from build123d import *

# Parameters (mm, degrees)
BOSS_EXTRUDE1_DEPTH = 2
SKETCH2_W           = 10
SKETCH2_H           = 30
CUT_EXTRUDE1_DEPTH  = 3
FILLET1_R           = 1
CUT_EXTRUDE2_REACH  = 4
SKETCH3_R           = 1.6


with BuildPart() as part:
    # Sketch1 → Boss-Extrude1 (new body)
    with BuildSketch(Plane(origin=(0, 0, 0), x_dir=(1, 0, 0), z_dir=(0, 1, 0))):
        with BuildLine():
            ThreePointArc((-49.7, -34.741676707), (-48.154415588, -35.654415588), (-47.241676707, -37.2))
            Line((-47.241676707, -37.2), (47.241676707, -37.2))
            ThreePointArc((47.241676707, -37.2), (48.154415588, -35.654415588), (49.7, -34.741676707))
            Line((49.7, -34.741676707), (49.7, 34.741676707))
            ThreePointArc((49.7, 34.741676707), (48.154415588, 35.654415588), (47.241676707, 37.2))
            Line((47.241676707, 37.2), (-47.241676707, 37.2))
            ThreePointArc((-47.241676707, 37.2), (-48.154415588, 35.654415588), (-49.7, 34.741676707))
            Line((-49.7, 34.741676707), (-49.7, -34.741676707))
        make_face()
    extrude(amount=BOSS_EXTRUDE1_DEPTH)

    # Sketch2 → Cut-Extrude1 (cut, through all)
    with BuildSketch(Plane(origin=(0, 2, 0), x_dir=(1, 0, 0), z_dir=(0, 1, 0))):
        with Locations((-34.7, 0)):
            Rectangle(SKETCH2_W, SKETCH2_H)
    extrude(amount=-CUT_EXTRUDE1_DEPTH, mode=Mode.SUBTRACT)

    # Fillet1
    fillet1_edges = [part.edges().sort_by_distance(p)[0] for p in [
        (-29.7, 1, -15),
        (-29.7, 1, 15),
        (-39.7, 1, 15),
        (-39.7, 1, -15),
    ]]
    fillet(fillet1_edges, radius=FILLET1_R)

    # Sketch3 → Cut-Extrude2 (cut, up to next)
    with BuildSketch(Plane(origin=(0, 2, 0), x_dir=(1, 0, 0), z_dir=(0, 1, 0)), mode=Mode.PRIVATE) as cut_extrude2_sk1:
        with Locations((-13.794673406, 16.290721811)):
            Circle(SKETCH3_R)
    cut_extrude2_tool1 = extrude(cut_extrude2_sk1.sketch, amount=-CUT_EXTRUDE2_REACH, mode=Mode.PRIVATE) & part.part
    add(cut_extrude2_tool1.solids().sort_by_distance((-13.794673, 2, -16.290722))[0], mode=Mode.SUBTRACT)
    # Sketch3 → Cut-Extrude2 (cut, up to next)
    with BuildSketch(Plane(origin=(0, 2, 0), x_dir=(1, 0, 0), z_dir=(0, 1, 0)), mode=Mode.PRIVATE) as cut_extrude2_sk2:
        with Locations((34.973326594, -9.541278189)):
            Circle(SKETCH3_R)
    cut_extrude2_tool2 = extrude(cut_extrude2_sk2.sketch, amount=-CUT_EXTRUDE2_REACH, mode=Mode.PRIVATE) & part.part
    add(cut_extrude2_tool2.solids().sort_by_distance((34.973327, 2, 9.541278))[0], mode=Mode.SUBTRACT)


solid = part.part
For this review, take the finished solid that the model builds, in its own axes (mm). A direction names the side the tool comes from. Give positions to 0.01 mm unless a question says otherwise; leave off trailing zeros. Loops run counter-clockwise (first coordinate to the right, second up) from the corner with the lowest first, then second, coordinate; pieces in that order, holes last. Notation, with made-up numbers: M 86.25,12.25 L 111.25,12.25 A19 ccw 111.25,49.25 Z; hole C 66,68.25 d3. An arc over 180 degrees is marked long. Answer as a JSON object with one key per item and string values. Group by question number.
Q1. Add section B-B on y = 1. Give the boundary of the cut face in (x, z), and give its area (3 significant figures).
Q2. For probe 1 along X at (y, z) = (0.5, -3.5); probe 2 along Z at (x, y) = (-31, 1.65); probe 3 along X at (y, z) = (0.45, 10.5), list the stretches that pass through material, from the lowest coordinate up. Write a range as [from, to].
Q3. Add section A-A on z = -9. Give the boundary of the cut face in (x, y), and give its area (3 significant figures).
Q4. Mouldability with a two-part tool opening along X and no side actions: class faces 3 (the flat face through (1, 1, -37.2)), 4 (the flat face through (-35, 1, -15)), 5 (the flat face through (49.7, 1, 0)), 6 (the cylindrical face through (-48.17, 0.99, 35.64)) as +X half, -X half, draft (parallel to the pull), parting line (faces both ways), or undercut.
Q5. Tool access review of faces 1 (the flat face through (-49.7, 1, 0)), 2 (the flat face through (-39.7, 1, 0)): name each direction out of +Z, -Z, +X, -X, +Y, -Y from which nothing blocks a thin tool from reaching the whole face with its end or side.
Checked values:
{
 "1": {"outline": "M -49.7,-34.74 A3.6 cw -47.24,-37.2 L 47.24,-37.2 A3.6 cw 49.7,-34.74 L 49.7,34.74 A3.6 cw 47.24,37.2 L -47.24,37.2 A3.6 cw -49.7,34.74 Z; hole M -39.7,-14 A1 ccw -38.7,-15 L -30.7,-15 A1 ccw -29.7,-14 L -29.7,14 A1 ccw -30.7,15 L -38.7,15 A1 ccw -39.7,14 Z; hole C -13.79,-16.29 d3.2; hole C 34.97,9.54 d3.2", "area": "7,060 mm²"},
 "2": {"probe 1": "[-49.7, -39.7], [-29.7, 49.7]", "probe 2": "[-37.2, -15], [15, 37.2]", "probe 3": "[-49.7, -39.7], [-29.7, 33.69], [36.25, 49.7]"},
 "3": {"outline": "M -49.7,0 L -39.7,0 L -39.7,2 L -49.7,2 Z; M -29.7,0 L 49.7,0 L 49.7,2 L -29.7,2 Z", "area": "179 mm²"},
 "4": {"face 3": "draft", "face 4": "undercut", "face 5": "+X half", "face 6": "-X half"},
 "5": {"face 1": "+Z, -Z, -X, +Y, -Y", "face 2": "+Y, -Y"}
}
